Could you check a few things on this drawing? It's one solid part, dimensions in mm from its lowest x, y, z. A direction names the side the tool comes from. Round coordinates to 2 decimals unless told otherwise and drop trailing zeros. Order: outer loops, then holes, each group sorted by start corner. A loop starts at its lowest first (then second) coordinate and runs counter-clockwise, first axis right, second up. Notation, with made-up numbers: (-2, 36) -> (53, 36) arc R9 ccw to (53, 48) -> close; hole circle Ø5 at (-17.75, -27.75). An arc over 180 degrees is marked (long way). Use a Markdown table: item, result. Add a question column.
(1) If I drill on probe 1 along X at (y, z) = (4.5, 19.5); probe 2 along X at (y, z) = (30, 16), over which ranges is the centre line in solid material (lowest first)?
(2) I'm going to push flat-ended pins straight in: P1, Ø3.5, axis at x = 4.5, y = 5, coming from the +Z side; P2, Ø8, axis at x = 17.5, y = 27.5, coming from the +Z side; P3, Ø2.5, axis at x = 4.6, y = 4.6, coming from the +Z side. Where does each tip first touch, or does it pass through?
(3) I want a section at C-C, the plane z = 26. Please give me the cut outline in (x, y), then the cut area to 3 significant figures.
(4) I want a section at A-A, the plane x = 17.6. Please give me the cut outline in (y, z).
(5) I want a section at B-B, the plane y = 4.6. Please give me the cut outline in (x, z), then the cut area to 3 significant figures.
(6) I want a section at D-D, the plane y = 25. Please give me the cut outline in (x, z), then the cut area to 3 significant figures.
(7) On a 3-axis mill with a long thin cutter (end or side, diameter ignored), from which of +Z, -Z, +X, -X, +Y, -Y can I reach the whole of each face in a straight line? I mean the marked faces 1 and 2. Say none if no direction works.
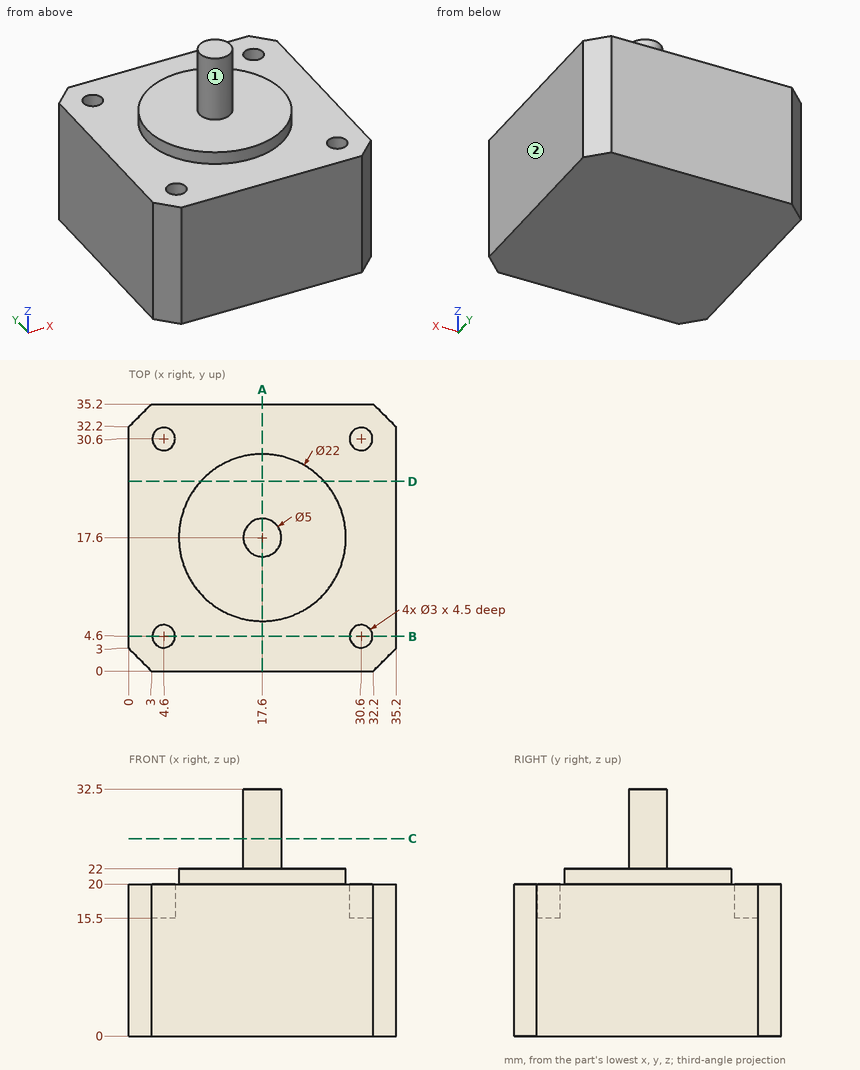
Taken from the geometry:
| question | item | result |
|---|---|---|
| 1 | probe 1 | x = 0 to 3.1, 6.1 to 29.1, 32.1 to 35.2 |
| 1 | probe 2 | x = 0 to 3.23, 5.97 to 29.23, 31.97 to 35.2 |
| 2 | P1 | stops at z = 20 |
| 2 | P2 | stops at z = 22 |
| 2 | P3 | stops at z = 15.5 |
| 3 | outline | circle Ø5 at (17.6, 17.6) |
| 3 | area | 19.6 mm2 |
| 4 | outline | (0, 0) -> (35.2, 0) -> (35.2, 20) -> (28.6, 20) -> (28.6, 22) -> (20.1, 22) -> (20.1, 32.5) -> (15.1, 32.5) -> (15.1, 22) -> (6.6, 22) -> (6.6, 20) -> (0, 20) -> close |
| 5 | outline | (0, 0) -> (35.2, 0) -> (35.2, 20) -> (32.1, 20) -> (32.1, 15.5) -> (29.1, 15.5) -> (29.1, 20) -> (6.1, 20) -> (6.1, 15.5) -> (3.1, 15.5) -> (3.1, 20) -> (0, 20) -> close |
| 5 | area | 677 mm2 |
| 6 | outline | (0, 0) -> (35.2, 0) -> (35.2, 20) -> (25.74, 20) -> (25.74, 22) -> (9.46, 22) -> (9.46, 20) -> (0, 20) -> close |
| 6 | area | 737 mm2 |
| 7 | face 1 | +Z |
| 7 | face 2 | +Z, -Z, +X, +Y, -Y |
